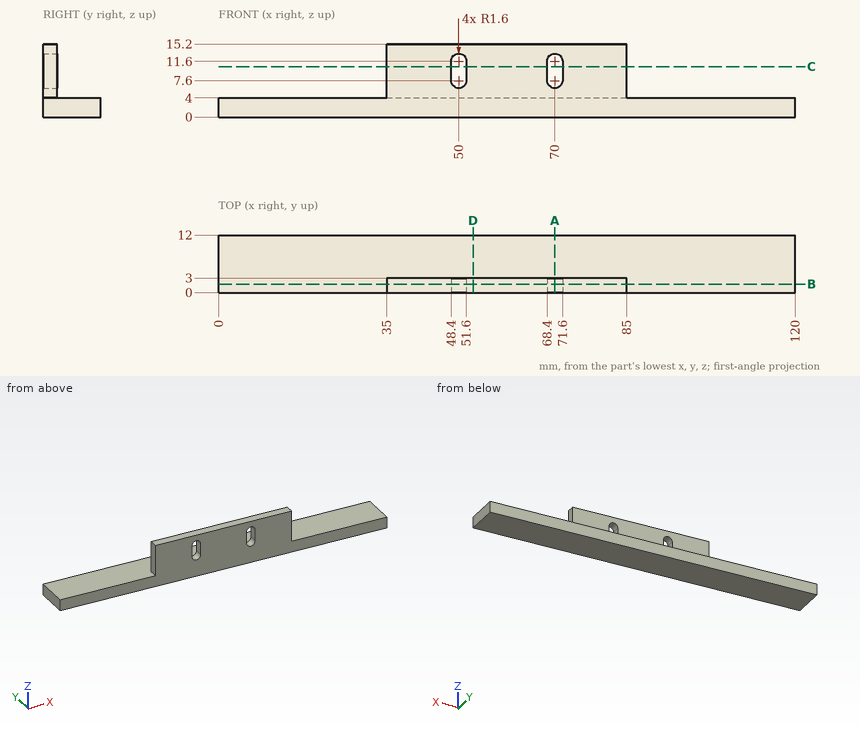
Can you work these out from the drawing? Everything is in mm from the part's minimum corner. Round coordinates to 2 decimals unless told otherwise and drop trailing zeros. Order: outer loops, then holes, each group sorted by start corner. A loop starts at its lowest first (then second) coordinate and runs counter-clockwise, first axis right, second up. Notation, with made-up numbers: (50, 15) -> (86, 15) arc R15 cw to (86, 24) -> close; hole circle Ø2 at (-31, -35). An arc over 180 degrees is marked (long way). Return JSON: item names as keys, results as strings. Group by question number.
1. I need wall thicknesses on line 1 (X direction, y = 2.5, z = 7.5); line 2 (X direction, y = 2.75, z = 7); line 3 (Y direction, x = 72.5, z = 5.75). Which ranges of each line are inside material? Lowest first, please. Write a range as [from, to].
2. Will these pins go through, and if not, where does the flat tip stop? pin 1 (2.5 mm diameter, centred on y = 2, z = 9.5, fed in from -X); pin 2 (0.9 mm diameter, centred on y = 2, z = 8, fed in from +X); pin 3 (9 mm diameter, centred on x = 55, z = 8, fed in from +Y).
3. If we section it at A-A, the plane x = 70: Write out the boundary of the cut face in (y, z), then the cut area to 3 significant figures.
4. If we section it at C-C, the plane z = 10.5: Write out the boundary of the cut face in (x, y).
5. If we section it at B-B, the plane y = 1.75: Write out the boundary of the cut face in (x, z), then the cut area to 3 significant figures.
6. If we section it at D-D, the plane x = 53: Write out the boundary of the cut face in (y, z).
Output values:
{
 "1": {"line 1": "[35, 48.4], [51.6, 68.4], [71.6, 85]", "line 2": "[35, 48.52], [51.48, 68.52], [71.48, 85]", "line 3": "[0, 3]"},
 "2": {"pin 1": "x = 35", "pin 2": "x = 85", "pin 3": "y = 12"},
 "3": {"outline": "(0, 0) -> (12, 0) -> (12, 4) -> (3, 4) -> (3, 6) -> (0, 6) -> close; (0, 13.2) -> (3, 13.2) -> (3, 15.2) -> (0, 15.2) -> close", "area": "60.0 mm²"},
 "4": {"outline": "(35, 0) -> (48.4, 0) -> (48.4, 3) -> (35, 3) -> close; (51.6, 0) -> (68.4, 0) -> (68.4, 3) -> (51.6, 3) -> close; (71.6, 0) -> (85, 0) -> (85, 3) -> (71.6, 3) -> close"},
 "5": {"outline": "(0, 0) -> (120, 0) -> (120, 4) -> (85, 4) -> (85, 15.2) -> (35, 15.2) -> (35, 4) -> (0, 4) -> close; hole (48.4, 7.6) arc R1.6 ccw to (51.6, 7.6) -> (51.6, 11.6) arc R1.6 ccw to (48.4, 11.6) -> close; hole (68.4, 7.6) arc R1.6 ccw to (71.6, 7.6) -> (71.6, 11.6) arc R1.6 ccw to (68.4, 11.6) -> close", "area": "998 mm²"},
 "6": {"outline": "(0, 0) -> (12, 0) -> (12, 4) -> (3, 4) -> (3, 15.2) -> (0, 15.2) -> close"}
}
